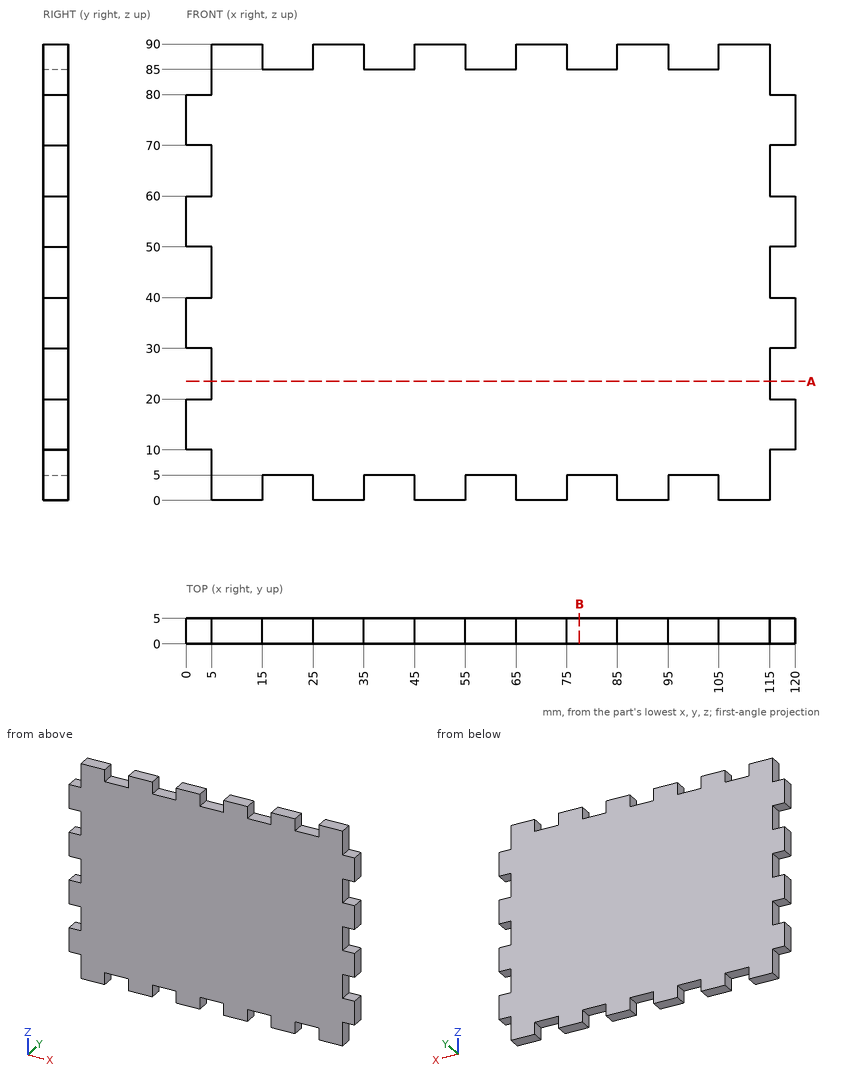
Answer from the drawing. Dimensions are ordinates in mm from the lowest x, y and z of the part. Give positions to 0.01 mm unless a question says otherwise; leave off trailing zeros. Order: outer loops, then holes, each group sorted by start corner. A loop starts at its lowest first (then second) coordinate and runs counter-clockwise, first axis right, second up. Notation, with made-up numbers: (66, -19) - (70, -19) arc R31 ccw to (70, 8) - close; hole circle Ø6 at (-2.5, -29.75). An arc over 180 degrees is marked (long way). One line per item, written item: value. Start each with the question number.
1. Each of these flat-tipped pins is pushed along its axis until it touches: pin 1 Ø2.5 at (x, y) = (116.5, 3.5) entering from -Z; pin 2 Ø2.5 at (y, z) = (2, 87.5) entering from +X; pin 3 Ø1.5 at (x, z) = (75.5, 76.5) entering from -Y; pin 4 Ø2.5 at (y, z) = (1.5, 88) entering from -X. Where does it stop, or does it pass through?
2. Section A-A, the plane z = 23.5 is taken. Write down the section's boundary in (x, y), then the cut area to 3 significant figures.
3. Section B-B, the plane x = 77.5 is taken. Write down the section's boundary in (y, z), then the cut area to 3 significant figures.
4. Consider line 1 (X direction, y = 4.6, z = 9.5); line 2 (Z direction, x = 37.5, y = 0.3). Determine where each line is inside the solid, lowest interval first.
Filled sheet:
1. pin 1: z = 10
1. pin 2: x = 115
1. pin 3: y = 0
1. pin 4: x = 5
2. outline: (5, 0) - (115, 0) - (115, 5) - (5, 5) - close
2. area: 550 mm²
3. outline: (0, 5) - (5, 5) - (5, 85) - (0, 85) - close
3. area: 400 mm²
4. line 1: 5 to 115
4. line 2: 5 to 85
